from build123d import *

# Parameters (mm, degrees)
ESQUISSE1_R      = 6
EXTRUSION1_DEPTH = 20
ESQUISSE2_W      = 4
ESQUISSE2_H      = 6.5
EXTRUSION2_DEPTH = 20


with BuildPart() as part:
    # Esquisse1 → Extrusion1 (new body)
    with BuildSketch(Plane.XY):
        Circle(ESQUISSE1_R)
    extrude(amount=EXTRUSION1_DEPTH)

    # Esquisse2 → Extrusion2 (cut)
    with BuildSketch(Plane(origin=(0, 0, 0), x_dir=(-1, 0, 0), z_dir=(0, 0, -1))):
        Rectangle(ESQUISSE2_W, ESQUISSE2_H)
    extrude(amount=-EXTRUSION2_DEPTH, mode=Mode.SUBTRACT)


solid = part.part
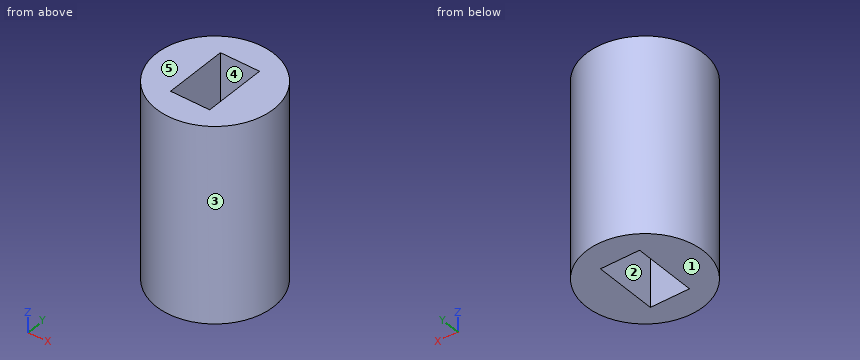
CAD build for the part. Positions are in the model's coordinates, mm. Face numbers are marked on the shaded views. A direction names the side the tool comes from. Round coordinates to 2 decimals unless told otherwise and drop trailing zeros. Write each loop counter-clockwise with the first axis right and the second up, starting at its lowest first coordinate (ties: lowest second). Pieces come first, ordered by that corner, then holes. Notation, with made-up numbers: M 20,-25.75 L 48,-25.75 A21 ccw 48,6.25 Z; hole C 51.5,85.25 d11. An arc over 180 degrees is marked long. Put each result on its own line as item: value. Start each with the question number.
1) 3-axis set-ups, long thin cutter, end or side, ignore diameter. For the marked faces 1 and 2: which of +Z, -Z, +X, -X, +Y, -Y reach the whole face in a straight line?
2) Saw through at A-A, the plane y = 0. Write the cut outline in (x, z).
3) Pull direction Y, two halves, no side cores. Call the marked faces 3, 4 and 5: pulls with the +Y half, pulls with the -Y half, needs draft (parallel to the pull), parting line crosses it, or undercut.
4) Saw through at B-B, the plane x = 0. Write the cut outline in (y, z).
5) Saw through at C-C, the plane z = 8.5. Write the cut outline in (x, y), and give its area (3 significant figures).
6) Drill centre lines: probe 1 along Y at (x, z) = (0, 9.25); probe 2 along X at (y, z) = (0.25, 13.5); probe 3 along X at (y, z) = (-1.75, 5). Where is each one in solid material? Low to high. Write a range as [from, to].
7) Saw through at D-D, the plane y = 4.5. Write the cut outline in (x, z).
8) Pin check, flat tips, straight feed: pin 1 Ø4 at (y, z) = (-0.5, 4.5) entering from -X; pin 2 Ø5 at (y, z) = (4, 12.5) entering from -X; pin 3 Ø5 at (y, z) = (-4.5, 4) entering from -X; pin 4 Ø2 at (x, z) = (-3.5, 17) entering from +Y. Stop position of each tip, or through.
Resolved:
1. face 1: -Z, +X, -X, +Y, -Y
1. face 2: +Z, -Z
2. outline: M -6,0 L -2,0 L -2,20 L -6,20 Z; M 2,0 L 6,0 L 6,20 L 2,20 Z
3. face 3: parting line crosses it
3. face 4: undercut
3. face 5: needs draft
4. outline: M -6,0 L -3.25,0 L -3.25,20 L -6,20 Z; M 3.25,0 L 6,0 L 6,20 L 3.25,20 Z
5. outline: C 0,0 d12; hole M -2,-3.25 L 2,-3.25 L 2,3.25 L -2,3.25 Z
5. area: 87.1 mm²
6. probe 1: [-6, -3.25], [3.25, 6]
6. probe 2: [-5.99, -2], [2, 5.99]
6. probe 3: [-5.74, -2], [2, 5.74]
7. outline: M -3.97,0 L 3.97,0 L 3.97,20 L -3.97,20 Z
8. pin 1: x = -6
8. pin 2: x = -5.81
8. pin 3: x = -5.66
8. pin 4: y = 5.45
